The figure shows three views and two pictorial views of one solid part (mm, origin at its lowest corner). Answer the questions. A direction names the side the tool comes from. Round coordinates to 2 decimals unless told otherwise and drop trailing zeros. Write each loop counter-clockwise with the first axis right and the second up, starting at its lowest first coordinate (ties: lowest second). Pieces come first, ordered by that corner, then holes. Notation, with made-up numbers: (10.25, 30.5) - (14.25, 30.5) arc R29 ccw to (14.25, 69.5) - close; hole circle Ø6 at (19.5, 16). An arc over 180 degrees is marked (long way). Answer as CSV lines item,"result". Start each with the question number.
Item 1: For a pull along X with two mould halves and no side action, classify the marked faces 3, 4 and 5 as pulls with the +X half, pulls with the -X half, needs draft (parallel to the pull), parting line crosses it, or undercut.
Item 2: Which of the six approach directions +Z, -Z, +X, -X, +Y, -Y give full straight-line access (tool end or side, diameter ignored) to the marked faces 1 and 2?
Item 3: A cutting plane is placed at A-A on x = 4.75. Determine the outline of the cut face in (y, z).
Item 4: A cutting plane is placed at C-C on z = 11.5. Determine the outline of the cut face in (x, y).
Item 5: Flat-ended cylindrical pins translate along their axes: pin 1 (1 mm diameter, centred on x = 7.5, y = 24, fed in from +Z) (1 decimal); pin 2 (4 mm diameter, centred on x = 5, y = 14.5, fed in from -Z); pin 3 (1 mm diameter, centred on y = 16.5, z = 12, fed in from -X); pin 4 (5 mm diameter, centred on y = 3, z = 6, fed in from -X). Find the tip coordinate at first contact, or state that the pin passes through.
Item 6: A cutting plane is placed at D-D on z = 3.5. Determine the outline of the cut face in (x, y).
Item 7: Straight lines are drawn through the part: line 1 along Z through (x, y) = (4.75, 21.5); line 2 along X through (y, z) = (14, 3.75); line 3 along X through (y, z) = (20.5, 8.25) (1 decimal). For each, find the intervals that lie inside material, in ascending order. Write a range as [from, to].
Item 8: A cutting plane is placed at B-B on y = 9.25. Determine the outline of the cut face in (x, z).
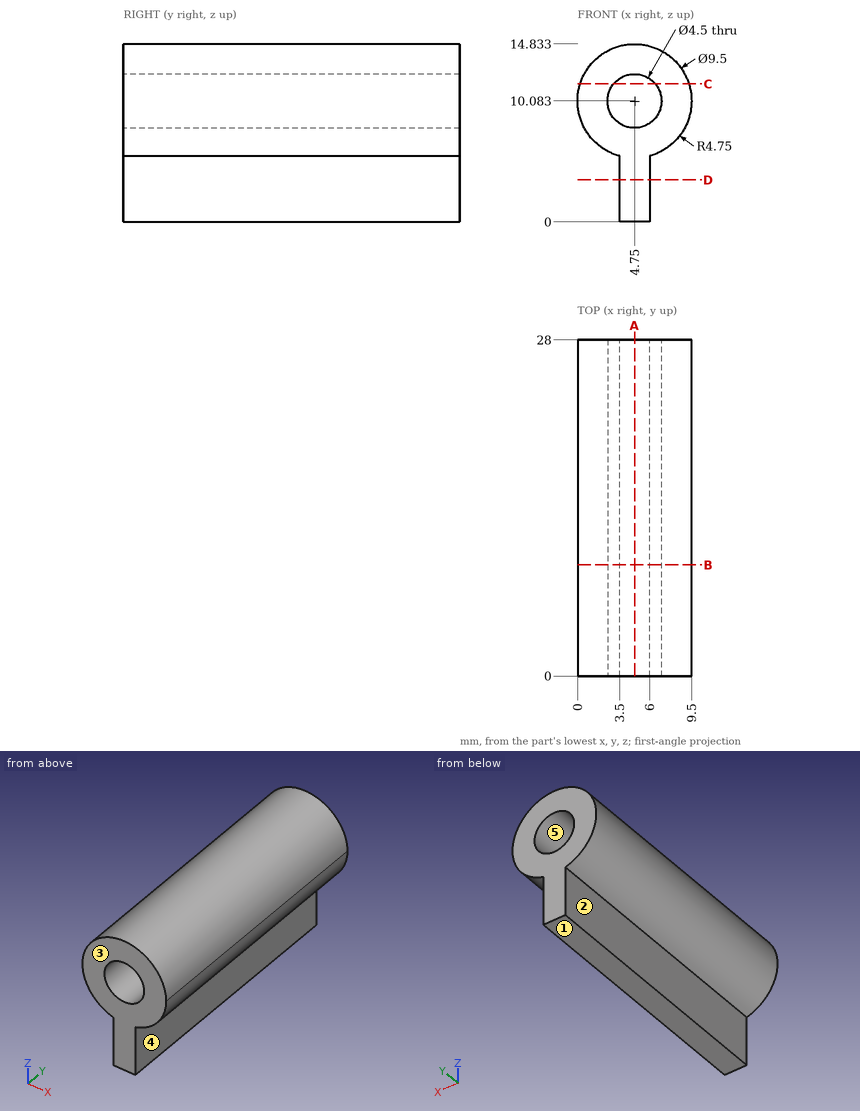
Geometry says:
1,face 3,"needs draft"
1,face 4,"pulls with the +X half"
1,face 5,"undercut"
2,face 1,"-Z, +X, -X, +Y, -Y"
2,face 2,"-Z, -X, +Y, -Y"
3,outline,"(0, 0) - (28, 0) - (28, 7.83) - (0, 7.83) - close; (0, 12.33) - (28, 12.33) - (28, 14.83) - (0, 14.83) - close"
4,outline,"(0.22, 0) - (3, 0) - (3, 28) - (0.22, 28) - close; (6.5, 0) - (9.28, 0) - (9.28, 28) - (6.5, 28) - close"
5,pin 1,"stops at z = 14.3"
5,pin 2,"stops at z = 0"
5,pin 3,"stops at x = 0.22"
5,pin 4,"stops at x = 0.27"
6,outline,"(3.5, 0) - (6, 0) - (6, 28) - (3.5, 28) - close"
7,line 1,"z = [0, 7.83], [12.33, 14.83]"
7,line 2,"x = [3.5, 6]"
7,line 3,"x = [0.4, 3.4], [6.1, 9.1]"
8,outline,"(3.5, 0) - (6, 0) - (6, 5.5) arc R4.75 ccw (long way) to (3.5, 5.5) - close; hole circle Ø4.5 at (4.75, 10.08)"
